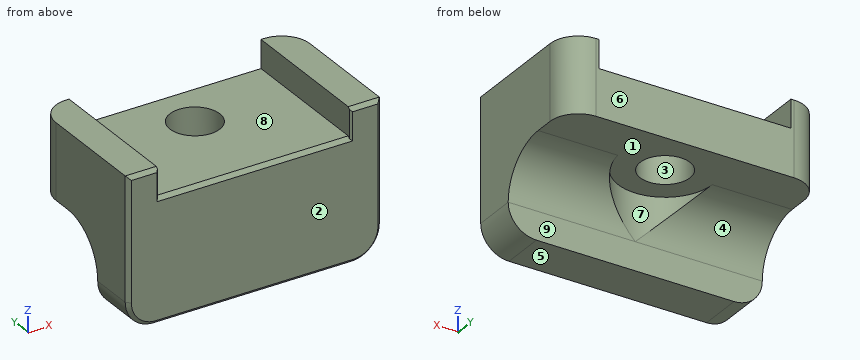
from build123d import *

# Parameters (mm, degrees)
BOSS_EXTRUDE1_DEPTH = 5
BOSS_EXTRUDE2_DEPTH = 10
FILLET1_R           = 5
FILLET2_R           = 3
SKETCH4_R           = 2.65
CUT_EXTRUDE1_DEPTH  = 22.708293346
SKETCH5_R           = 5
CUT_EXTRUDE2_DEPTH  = 22.708293346
CHAMFER1_SIZE       = 0.4
MOVE_START          = -10.2
MOVE_FACE1_DEPTH    = 20.4


with BuildPart() as part:
    # Sketch2 → Boss-Extrude1 (new body)
    with BuildSketch(Plane(origin=(0, 0, 0), x_dir=(1, 0, 0), z_dir=(0, 1, 0))):
        Polygon((-10, 10), (-10, 7), (-13.5, 7), (-13.5, 23), (13.5, 23), (13.5, 7), (10, 7), (10, 10), align=None)
    extrude(amount=BOSS_EXTRUDE1_DEPTH)

    # Sketch3 → Boss-Extrude2 (add)
    with BuildSketch(Plane(origin=(0, 5, 0), x_dir=(1, 0, 0), z_dir=(0, 1, 0))):
        Polygon((10, 7), (13.5, 7), (13.5, 15), (-13.5, 15), (-13.5, 7), (-10, 7), (-10, 10), (10, 10), align=None)
    extrude(amount=BOSS_EXTRUDE2_DEPTH)

    # Fillet1
    fillet1_edges = [part.edges().sort_by_distance(p)[0] for p in [
        (0, 5, -15),
    ]]
    fillet(fillet1_edges, radius=FILLET1_R)

    # Fillet2
    fillet2_edges = [part.edges().sort_by_distance(p)[0] for p in [
        (-13.5, 2.5, -23),
        (13.5, 2.5, -23),
        (-13.5, 15, -11),
        (13.5, 15, -11),
    ]]
    fillet(fillet2_edges, radius=FILLET2_R)

    # Sketch4 → Cut-Extrude1 (cut, through all)
    with BuildSketch(Plane(origin=(0, 0, -15), x_dir=(-1, 0, 0), z_dir=(0, 0, -1))):
        with Locations((0, 10)):
            Circle(SKETCH4_R)
    extrude(amount=-CUT_EXTRUDE1_DEPTH, mode=Mode.SUBTRACT)

    # Sketch5 → Cut-Extrude2 (cut, through all)
    with BuildSketch(Plane(origin=(0, 0, -15), x_dir=(-1, 0, 0), z_dir=(0, 0, -1))):
        with Locations((0, 10)):
            Circle(SKETCH5_R)
    extrude(amount=CUT_EXTRUDE2_DEPTH, mode=Mode.SUBTRACT)

    # Chamfer1
    chamfer1_edges = [part.edges().sort_by_distance(p)[0] for p in [
        (13.5, 0, -13.5),
        (11.75, 0, -7),
        (10, 0, -8.5),
        (-13.5, 0, -13.5),
        (0, 0, -23),
        (12.621320344, 0, -22.121320344),
        (-12.621320344, 0, -22.121320344),
        (0, 0, -10),
        (-10, 0, -8.5),
        (-11.75, 0, -7),
    ]]
    chamfer(chamfer1_edges, length=CHAMFER1_SIZE)

    # Move Face1: read off the stored shape, not the designer's step
    # Move Face1 outline → Move Face1 (cut)
    with BuildSketch(Plane.YZ.offset(MOVE_START)):
        Polygon((0.4, -10), (15, -10), (15, -7), (0.4, -7), (0.2, -7.2), (0.2, -10.2), align=None)
    extrude(amount=MOVE_FACE1_DEPTH, mode=Mode.SUBTRACT)


solid = part.part
Model file for the job. Use its own axes, mm. Face numbers are marked on the shaded views. A direction names the side the tool comes from. Give positions to 0.01 mm unless a question says otherwise; leave off trailing zeros. Order: outer loops, then holes, each group sorted by start corner. A loop starts at its lowest first (then second) coordinate and runs counter-clockwise, first axis right, second up. Notation, with made-up numbers: (41, 75.5) - (71, 75.5) arc R21 cw to (71, 94.5) - close; hole circle Ø3 at (56, 50.25). An arc over 180 degrees is marked (long way). Write item = value, one per line. Start each with the question number.
1. Two-plate mould, pull along Y, no slides. Class the marked faces 1, 2, 3 and 4: pulls with the +Y half, pulls with the -Y half, needs draft (parallel to the pull), parting line crosses it, or undercut.
2. Cut at B-B, the plane y = 1.5. List the corners of the cut face in (x, z), and give its area (3 significant figures).
3. Cut at C-C, the plane z = -14. List the corners of the cut face in (x, y), and give its area (3 significant figures).
4. Probe line 1 along X through (y, z) = (10, -13.9); line 2 along Y through (x, z) = (0, -13.7); line 3 along Z through (x, y) = (3.5, 14.5). List the from-to ranges inside material, lowest first.
5. Drop flat-ended pins along their axis: P1, Ø3, axis at x = 0, y = 13.5, coming from the -Z side; P2, Ø5, axis at x = 7.5, y = 9.5, coming from the +Z side; P3, Ø1.5, axis at y = 9, z = -16.5, coming from the +X side; P4, Ø1.5, axis at x = 2, z = -21, coming from the +Y side. Give the stop position or say it passes through.
6. Cut at D-D, the plane y = 11.5. List the corners of the cut face in (x, z), and give its area (3 significant figures).
7. Cut at A-A, the plane z = -8. List the corners of the cut face in (x, y).
8. Which spindle directions (+Z, -Z, +X, -X, +Y, -Y) get a long thin tool onto all of the face, cutting with end or side? Do the marked faces 5, 6, 7, 8 and 9. Say none if no direction does.
Taken from the geometry:
q1.face_1 = needs draft
q1.face_2 = pulls with the -Y half
q1.face_3 = undercut
q1.face_4 = pulls with the +Y half
q2.outline = (-13.5, -20) arc R3 ccw to (-10.5, -23) - (10.5, -23) arc R3 ccw to (13.5, -20) - (13.5, -7) - (10.2, -7) - (10.2, -10) - (-10.2, -10) - (-10.2, -7) - (-13.5, -7) - close
q2.area = 367 mm²
q3.outline = (-13.5, 0.4) - (-13.1, 0) - (13.1, 0) - (13.5, 0.4) - (13.5, 12) arc R3 ccw to (10.5, 15) - (-10.5, 15) arc R3 ccw to (-13.5, 12) - close; hole circle Ø5.3 at (0, 10)
q3.area = 379 mm²
q4.line_1 = -13.5 to -2.65, 2.65 to 13.5
q4.line_2 = 0 to 7.35, 12.65 to 15
q4.line_3 = -15 to -10
q5.P1 = -15
q5.P2 = -10
q5.P3 = through
q5.P4 = 5
q6.outline = (-13.5, -15) - (-2.18, -15) - (-2.18, -10) - (-10.2, -10) - (-10.2, -7) - (-13.5, -7) - close; (2.18, -15) - (13.5, -15) - (13.5, -7) - (10.2, -7) - (10.2, -10) - (2.18, -10) - close
q6.area = 133 mm²
q7.outline = (-13.5, 0.4) - (-13.1, 0) - (-10.4, 0) - (-10.2, 0.2) - (-10.2, 15) - (-10.5, 15) arc R3 ccw to (-13.5, 12) - close; (10.2, 0.2) - (10.4, 0) - (13.1, 0) - (13.5, 0.4) - (13.5, 12) arc R3 ccw to (10.5, 15) - (10.2, 15) - close
q8.face_5 = -Z, +X, -X, +Y, -Y
q8.face_6 = +Z, -Z, +X, -X, +Y
q8.face_7 = -Z, +Y
q8.face_8 = +Z, +Y, -Y
q8.face_9 = -Z, +X, -X, +Y
